Input: part model. Units: mm. Frame: model coordinates. A direction names the side the tool comes from. Round coordinates to 2 decimals unless told otherwise and drop trailing zeros. Write each loop counter-clockwise with the first axis right and the second up, starting at its lowest first coordinate (ties: lowest second). Pieces come first, ordered by that corner, then holes. Notation, with made-up numbers: (46.25, 32) -> (54.25, 32) arc R34 cw to (54.25, 68) -> close; hole circle Ø5 at (-1.75, 7.5). An arc over 180 degrees is marked (long way). Write item = value, one per line.
```python
from build123d import *

# Parameters (mm, degrees)
SKETCH1_R           = 1.75
BOSS_EXTRUDE1_DEPTH = 5
SKETCH2_R           = 1.75
SKETCH2_R_2         = 6.4
CUT_EXTRUDE1_DEPTH  = 10
FILLET1_R           = 1


with BuildPart() as part:
    # Sketch1 → Boss-Extrude1 (new body)
    # profile 1 of 4: a face of its own
    with BuildSketch(Plane(origin=(0, 0, 0), x_dir=(1, 0, 0), z_dir=(0, 1, 0))):
        Polygon((50, 25), (0, 25), (0, 15), (10, 0), (26, 0), (36, 15), (50, 15), align=None)
        with Locations(Location((13, 5, 0), (0, 0, 270))):
            Circle(SKETCH1_R, mode=Mode.SUBTRACT)
        with Locations(Location((23, 5, 0), (0, 0, 270))):
            Circle(SKETCH1_R, mode=Mode.SUBTRACT)
    # profile 2 of 4: a face of its own
    with BuildSketch(Plane(origin=(0, 0, 0), x_dir=(1, 0, 0), z_dir=(0, 1, 0))):
        Polygon((10, 45), (0, 33.819660113), (0, 25), (50, 25), (50, 35), (36, 35), (26, 45), align=None)
    # profile 3 of 4: a face of its own
    with BuildSketch(Plane(origin=(0, 0, 0), x_dir=(1, 0, 0), z_dir=(0, 1, 0))):
        Polygon((10, 45), (0, 33.819660113), (0, 25), (50, 25), (50, 35), (36, 35), (26, 45), align=None)
    # profile 4 of 4: a face of its own
    with BuildSketch(Plane(origin=(0, 0, 0), x_dir=(1, 0, 0), z_dir=(0, 1, 0))):
        Polygon((10, 45), (0, 33.819660113), (0, 25), (50, 25), (50, 35), (36, 35), (26, 45), align=None)
    extrude(amount=BOSS_EXTRUDE1_DEPTH)

    # Sketch2 → Cut-Extrude1 (cut)
    with BuildSketch(Plane(origin=(0, 0, 0), x_dir=(-1, 0, 0), z_dir=(0, -1, 0))):
        with Locations(Location((-4.8, 24.409830056, 0), (0, 0, 90))):
            Circle(SKETCH2_R)
        with Locations(Location((-35.8, 24.409830056, 0), (0, 0, 90))):
            Circle(SKETCH2_R_2)
    extrude(amount=-CUT_EXTRUDE1_DEPTH, mode=Mode.SUBTRACT)

    # Fillet1
    fillet1_edges = [part.edges().sort_by_distance(p)[0] for p in [
        (35.8, 5, -18.009830056),
    ]]
    fillet(fillet1_edges, radius=FILLET1_R)


solid = part.part
```
1) Line query: L1, parallel to X at y = 3.15, z = -5; L2, parallel to X at y = 3.35, z = -23; L3, parallel to Z at x = 41, y = 1.3. Output: solid intervals per line, ascending. Write a range as from..to.
Solutions:
L1 = 6.67..11.25, 14.75..21.25, 24.75..29.33
L2 = 0..3.76, 5.84..29.56, 42.04..50
L3 = -35..-28.14, -20.68..-15
2) Cut plane C-C (z = -5). Return the cut outline in (x, y).
Solutions:
outline = (6.67, 0) -> (11.25, 0) -> (11.25, 5) -> (6.67, 5) -> close; (14.75, 0) -> (21.25, 0) -> (21.25, 5) -> (14.75, 5) -> close; (24.75, 0) -> (29.33, 0) -> (29.33, 5) -> (24.75, 5) -> close
3) Access query for faces 1 (the face through (24.735, 2.465, -5.228)), 2 (the face through (43, 2, -15)), 3 (the face through (43, 2, -35)). Directions: +Z, -Z, +X, -X, +Y, -Y. A direction counts if a zero-diameter tool reaches every point of the face in a straight line with its end or side. Return the directions, or none.
Solutions:
face_1 = +Y, -Y
face_2 = +Z, +X, +Y, -Y
face_3 = -Z, +X, +Y, -Y
4) Draft query along Z for faces 4 (the face through (0, 2, -25)), 5 (the face through (18, 2, -45)), 6 (the face through (18, 2, 0)), 7 (the face through (3.735, 2.465, -23.021)). Return one class per face: +Z half, -Z half, draft (parallel to the pull), parting line (faces both ways), or undercut.
Solutions:
face_4 = draft
face_5 = -Z half
face_6 = +Z half
face_7 = undercut
5) Cut plane B-B (y = 2.2). Return the cut outline in (x, z), and give its area (3 significant figures).
Solutions:
outline = (0, -33.82) -> (10, -45) -> (26, -45) -> (36, -35) -> (50, -35) -> (50, -15) -> (36, -15) -> (26, 0) -> (10, 0) -> (0, -15) -> close; hole circle Ø3.5 at (4.8, -24.41); hole circle Ø3.5 at (13, -5); hole circle Ø3.5 at (23, -5); hole circle Ø12.8 at (35.8, -24.41)
area = 1,490 mm^2
6) First-contact query: P1, Ø1, axis at y = 3, z = -5.5, coming from the -X side. Flat tip, straight axial feed; report the tip coordinate or a pass-through.
Solutions:
P1 = 6
7) Cut plane A-A (x = 13). Return the cut outline in (y, z).
Solutions:
outline = (0, -45) -> (5, -45) -> (5, -6.75) -> (0, -6.75) -> close; (0, -3.25) -> (5, -3.25) -> (5, 0) -> (0, 0) -> close
8) Cut plane D-D (x = 6). Return the cut outline in (y, z), and give its area (3 significant figures).
Solutions:
outline = (0, -40.53) -> (5, -40.53) -> (5, -25.68) -> (0, -25.68) -> close; (0, -23.14) -> (5, -23.14) -> (5, -6) -> (0, -6) -> close
area = 160 mm^2
